```python
from build123d import *

# Parameters (mm, degrees)
SKETCH1_R           = 50
BOSS_EXTRUDE1_DEPTH = 12
SKETCH3_R           = 40.1
CUT_EXTRUDE1_DEPTH  = 2
SKETCH4_R           = 39
CUT_EXTRUDE2_DEPTH  = 9
SKETCH6_W           = 24
SKETCH6_H           = 7
CUT_EXTRUDE4_DEPTH  = 61
SKETCH7_R           = 3
CUT_EXTRUDE5_DEPTH  = 61
CIRPATTERN1_COUNT   = 5


with BuildPart() as part:
    # Sketch1 → Boss-Extrude1 (new body)
    with BuildSketch(Plane(origin=(0, 0, 0), x_dir=(1, 0, 0), z_dir=(0, 1, 0))):
        with Locations(Location((0, 0, 0), (0, 0, 270))):
            Circle(SKETCH1_R)
    extrude(amount=BOSS_EXTRUDE1_DEPTH)

    # Sketch3 → Cut-Extrude1 (cut)
    with BuildSketch(Plane(origin=(0, 12, 0), x_dir=(1, 0, 0), z_dir=(0, 1, 0))):
        with Locations(Location((0, 0, 0), (0, 0, 270))):
            Circle(SKETCH3_R)
    extrude(amount=-CUT_EXTRUDE1_DEPTH, mode=Mode.SUBTRACT)

    # Sketch4 → Cut-Extrude2 (cut)
    with BuildSketch(Plane(origin=(0, 10, 0), x_dir=(1, 0, 0), z_dir=(0, 1, 0))):
        with Locations(Location((0, 0, 0), (0, 0, 270))):
            Circle(SKETCH4_R)
    extrude(amount=-CUT_EXTRUDE2_DEPTH, mode=Mode.SUBTRACT)

    # Sketch6 → Cut-Extrude4 (cut)
    with BuildSketch(Plane.XY):
        with Locations((0, 4.5)):
            Rectangle(SKETCH6_W, SKETCH6_H)
    extrude(amount=-CUT_EXTRUDE4_DEPTH, mode=Mode.SUBTRACT)

    # Sketch7 → Cut-Extrude5 (cut)
    with BuildSketch(Plane.YX):
        with Locations((5, 0)):
            Circle(SKETCH7_R)
    cut_extrude5 = extrude(amount=-CUT_EXTRUDE5_DEPTH, mode=Mode.SUBTRACT)

    # CirPattern1: Cut-Extrude5 ×5 about axis
    cirpattern1_axis = Axis((0, -0.6, 0), (0, 1, 0))
    for i in range(1, CIRPATTERN1_COUNT):
        add(cut_extrude5.rotate(cirpattern1_axis, i * 360 / CIRPATTERN1_COUNT), mode=Mode.SUBTRACT)


solid = part.part
```
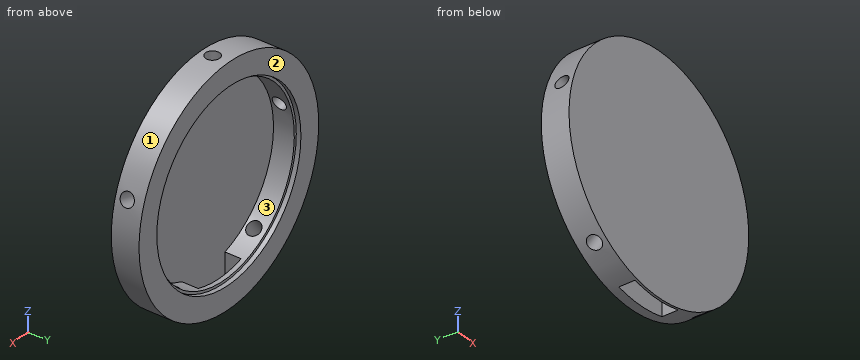
Input: part model. Units: mm. Frame: model coordinates. Face numbers are marked on the shaded views. Round coordinates to 2 decimals unless told otherwise and drop trailing zeros. Order: outer loops, then holes, each group sorted by start corner. A loop starts at its lowest first (then second) coordinate and runs counter-clockwise, first axis right, second up. Notation, with made-up numbers: (73, 6.25) - (112, 6.25) arc R35 cw to (112, 38.25) - close; hole circle Ø3 at (10, 18.5). An arc over 180 degrees is marked (long way). Answer in a Markdown table with one row per item.
Item 1: Section query D-D (x = -33). Return the cut outline in (y, z).
Model answer:
| item | result |
|---|---|
| outline | (0, -37.56) - (12, -37.56) - (12, -22.78) - (10, -22.78) - (10, -20.78) - (1, -20.78) - (1, 20.78) - (10, 20.78) - (10, 22.78) - (12, 22.78) - (12, 37.56) - (0, 37.56) - close |
Item 2: Section query C-C (y = 5). Return the cut outline in (x, z).
Model answer:
| item | result |
|---|---|
| outline | (-48.39, 12.57) arc R50 ccw to (-31.76, -38.61) - (-25.28, -29.69) arc R39 cw to (-37.91, 9.16) - close; (-46.54, 18.28) - (-36.05, 14.87) arc R39 cw to (-3, 38.88) - (-3, 49.91) arc R50 ccw to start; (-26.91, -42.14) arc R50 ccw to (-12, -48.54) - (-12, -37.11) arc R39 cw to (-20.43, -33.22) - close; (3, 38.88) arc R39 cw to (36.05, 14.87) - (46.54, 18.28) arc R50 ccw to (3, 49.91) - close; (12, -48.54) arc R50 ccw to (26.91, -42.14) - (20.43, -33.22) arc R39 cw to (12, -37.11) - close; (25.28, -29.69) - (31.76, -38.61) arc R50 ccw to (48.39, 12.57) - (37.91, 9.16) arc R39 cw to start |
Item 3: Line query: line 1 (X direction, y = 9.5, z = 1); line 2 (Y direction, x = 0, z = 43); line 3 (X direction, y = 10.7, z = 0). Output: solid intervals per line, ascending.
Model answer:
| item | result |
|---|---|
| line 1 | x = -49.99 to -38.99, 38.99 to 49.99 |
| line 2 | y = 0 to 2, 8 to 12 |
| line 3 | x = -50 to -40.1, 40.1 to 50 |
Item 4: Mould query, pull axis Z, two halves, no side actions, for the marked faces 1, 2 and 3. Classes: released by +Z, released by -Z, zero draft, split by the parting line, or undercut.
Model answer:
| item | result |
|---|---|
| face 1 | split by the parting line |
| face 2 | zero draft |
| face 3 | undercut |
Item 5: Section query B-B (z = 0). Return the cut outline in (x, y).
Model answer:
| item | result |
|---|---|
| outline | (-50, 0) - (50, 0) - (50, 12) - (40.1, 12) - (40.1, 10) - (39, 10) - (39, 1) - (-39, 1) - (-39, 10) - (-40.1, 10) - (-40.1, 12) - (-50, 12) - close |
Item 6: Pin query (flat end, axial travel): pin 1 (7 mm diameter, centred on x = 0, y = 5, fed in from -Z); pin 2 (3 mm diameter, centred on x = -19, y = 5, fed in from -Z); pin 3 (5 mm diameter, centred on x = 21.5, z = 12, fed in from +Y). Return the tip coordinate at first contact, or that it passes through.
Model answer:
| item | result |
|---|---|
| pin 1 | stops at z = -50 |
| pin 2 | stops at z = -46.84 |
| pin 3 | stops at y = 1 |
Item 7: Section query A-A (x = 0). Return the cut outline in (y, z).
Model answer:
| item | result |
|---|---|
| outline | (0, -50) - (1, -50) - (1, 39) - (2, 39) - (2, 50) - (0, 50) - close; (8, -50) - (12, -50) - (12, -40.1) - (10, -40.1) - (10, -39) - (8, -39) - close; (8, 39) - (10, 39) - (10, 40.1) - (12, 40.1) - (12, 50) - (8, 50) - close |
